Check sheet for the modelled part. Datum: model origin and axes. Units: mm. Face numbers are marked on the shaded views. A direction names the side the tool comes from. Round coordinates to 2 decimals unless told otherwise and drop trailing zeros. Loops run counter-clockwise (first coordinate to the right, second up) from the corner with the lowest first, then second, coordinate; pieces in that order, holes last. Notation, with made-up numbers: (75, 79.25) - (123, 79.25) arc R7 cw to (123, 89.25) - close; hole circle Ø2 at (69.25, 44). An arc over 180 degrees is marked (long way). Put each result on its own line as item: value. Start each with the question number.
```python
from build123d import *

# Parameters (mm, degrees)
F0_R     = 1.3
F0_R_2   = 1.85
F0_W     = 10
F0_H     = 18
F0_R_3   = 1.5
F1_DEPTH = 3
F2_DEPTH = 8
F3_D     = 5.5
F3_DEPTH = 3
F3_TIP   = 1.6523667023


with BuildPart() as f1:
    # F0 (on Front) → F1 (new body)
    with BuildSketch(Plane.XZ):
        Polygon((0, 3), (-10.5, 3), (-10.5, -5), (5, -5), (5, 13), (15, 13), (15, -5), (51.5, -5), (51.5, 12.5), (16, 12.5), (16, 50.0543485135), (0, 50.0543485135), align=None)
        with Locations((-6.5, -1)):
            Circle(F0_R, mode=Mode.SUBTRACT)
        with Locations((26.5, -1)):
            Circle(F0_R, mode=Mode.SUBTRACT)
        with Locations((47.5, 8.5)):
            Circle(F0_R_2, mode=Mode.SUBTRACT)
        with Locations((4, 45.5)):
            Circle(F0_R_2, mode=Mode.SUBTRACT)
        with Locations((10, 4)):
            Rectangle(F0_W, F0_H)
        with Locations((10, 1)):
            Circle(F0_R_3, mode=Mode.SUBTRACT)
        with Locations((10, 7)):
            Circle(F0_R_3, mode=Mode.SUBTRACT)
    extrude(amount=-F1_DEPTH)

    # F0 (on Front) → F2 (join)
    with BuildSketch(Plane.XZ):
        with Locations((10, 4)):
            Rectangle(F0_W, F0_H)
        with Locations((10, 1)):
            Circle(F0_R_3, mode=Mode.SUBTRACT)
        with Locations((10, 7)):
            Circle(F0_R_3, mode=Mode.SUBTRACT)
    extrude(amount=-F2_DEPTH)

    # F3
    with Locations(Plane.XZ):
        with Locations((10, 7), (10, 1)):
            Hole(F3_D / 2, depth=F3_DEPTH)
            with Locations((0, 0, -(F3_DEPTH + F3_TIP / 2))):  # 118° drill point
                Cone(0, F3_D / 2, F3_TIP, mode=Mode.SUBTRACT)


solid = f1.part
```
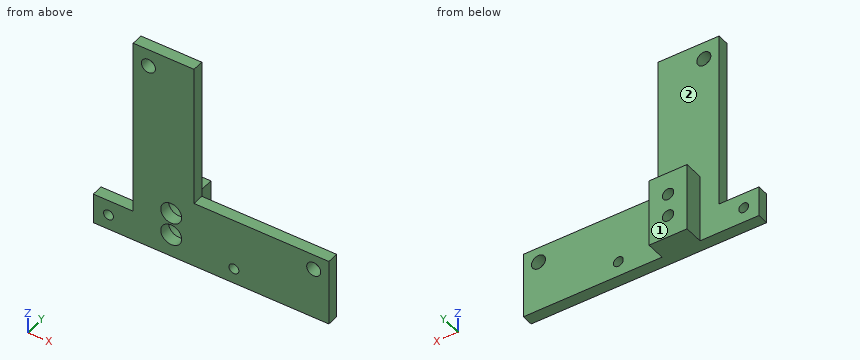
Q1. Cross-section at D-D on x = 10. Enter the section's corners in (y, z).
Q2. Depth check by flat-ended pin: pin 1 Ø4.5 at (x, z) = (10, 7) entering from -Y; pin 2 Ø4 at (x, z) = (10, 7) entering from -Y; pin 3 Ø1 at (y, z) = (5.5, 12) entering from +X; pin 4 Ø1.8 at (x, z) = (10, 1) entering from +Y. Enter the tip coordinate at first touch or a pass-through.
Q3. Cross-section at C-C on z = 45.5. Enter the section's corners in (x, y).
Q4. Set-up check for the marked faces 1 and 2: record each of +Z, -Z, +X, -X, +Y, -Y from which the full face is reachable in a straight line by a thin tool's end or side.
Q5. Material ranges on line 1 (Z direction, x = 10, y = 0.7); line 2 (Z direction, x = 10, y = 6.75); line 3 (X direction, y = 1.55, z = 7), recorded low to high. Write a range as from..to.
Q6. Cross-section at B-B on y = 0.75. Enter the section's corners in (x, z), and give its area (3 significant figures).
Q7. Cross-section at A-A on x = -6.5. Enter the section's corners in (y, z).
Answer list:
1. outline: (0, -5) - (8, -5) - (8, -0.5) - (3.75, -0.5) - (3, -1.75) - (0, -1.75) - close; (0, 3.75) - (3, 3.75) - (3.75, 2.5) - (8, 2.5) - (8, 5.5) - (3.75, 5.5) - (3, 4.25) - (0, 4.25) - close; (0, 9.75) - (3, 9.75) - (3.75, 8.5) - (8, 8.5) - (8, 13) - (3, 13) - (3, 50.05) - (0, 50.05) - close
2. pin 1: stops at y = 3.3
2. pin 2: stops at y = 3.45
2. pin 3: stops at x = 15
2. pin 4: passes through
3. outline: (0, 0) - (2.15, 0) - (2.15, 3) - (0, 3) - close; (5.85, 0) - (16, 0) - (16, 3) - (5.85, 3) - close
4. face 1: +Z, -Z, +X, -X, +Y
4. face 2: +Z, +Y
5. line 1: z = -5..-1.75, 3.75..4.25, 9.75..50.05
5. line 2: z = -5..-0.5, 2.5..5.5, 8.5..13
5. line 3: x = 0..7.25, 12.75..46.42, 48.58..51.5
6. outline: (-10.5, -5) - (51.5, -5) - (51.5, 12.5) - (16, 12.5) - (16, 50.05) - (0, 50.05) - (0, 3) - (-10.5, 3) - close; hole circle Ø2.6 at (-6.5, -1); hole circle Ø3.7 at (4, 45.5); hole circle Ø5.5 at (10, 1); hole circle Ø5.5 at (10, 7); hole circle Ø2.6 at (26.5, -1); hole circle Ø3.7 at (47.5, 8.5)
6. area: 1,510 mm2
7. outline: (0, -5) - (3, -5) - (3, -2.3) - (0, -2.3) - close; (0, 0.3) - (3, 0.3) - (3, 3) - (0, 3) - close
